```python
from build123d import *

# Parameters (mm, degrees)
F0_R     = 1.27
F1_DEPTH = 0.1


with BuildPart() as f1:
    # F0 (on Top) → F1 (new body)
    with BuildSketch(Plane.XY):
        with BuildLine():
            Line((0, 25.4), (0, 0))
            Line((0, 0), (44.45, 0))
            Line((44.45, 0), (88.9, 0))
            Line((88.9, 0), (88.9, 50.8))
            Line((88.9, 50.8), (57.15, 50.8))
            ThreePointArc((57.15, 50.8), (44.45, 44.45), (31.75, 50.8))
            Line((31.75, 50.8), (0, 50.8))
            Line((0, 50.8), (0, 25.4))
        make_face()
        with Locations((12.7, 9.525)):
            Circle(F0_R, mode=Mode.SUBTRACT)
        with BuildLine():
            ThreePointArc((13.97, 25.4), (12.7, 24.13), (11.43, 25.4))
            ThreePointArc((11.43, 25.4), (12.7, 26.67), (13.97, 25.4))
        make_face(mode=Mode.SUBTRACT)
        with Locations((31.75, 25.4)):
            Circle(F0_R, mode=Mode.SUBTRACT)
        with BuildLine():
            ThreePointArc((45.72, 12.7), (45.348026, 11.801974), (44.45, 11.43))
            ThreePointArc((44.45, 11.43), (43.551974, 13.598026), (45.72, 12.7))
        make_face(mode=Mode.SUBTRACT)
        with Locations((76.2, 9.525)):
            Circle(F0_R, mode=Mode.SUBTRACT)
        with Locations((44.45, 25.4)):
            Circle(F0_R, mode=Mode.SUBTRACT)
        with Locations((57.15, 25.4)):
            Circle(F0_R, mode=Mode.SUBTRACT)
        with Locations((76.2, 25.4)):
            Circle(F0_R, mode=Mode.SUBTRACT)
        with Locations((12.7, 41.275)):
            Circle(F0_R, mode=Mode.SUBTRACT)
        with Locations((44.45, 38.1)):
            Circle(F0_R, mode=Mode.SUBTRACT)
        with Locations((76.2, 41.275)):
            Circle(F0_R, mode=Mode.SUBTRACT)
    extrude(amount=F1_DEPTH)


solid = f1.part
```
Verification items for the finished model (mm, model axes). Round coordinates to 2 decimals unless told otherwise and drop trailing zeros. Order: outer loops, then holes, each group sorted by start corner. A loop starts at its lowest first (then second) coordinate and runs counter-clockwise, first axis right, second up.
1) Cross-section at B-B, the plane x = 76.2. Record the cut outline in (y, z) (3 decimals), plus the area to 3 significant figures.
Geometry says:
outline: (0, 0) - (8.255, 0) - (8.255, 0.1) - (0, 0.1) - close; (10.795, 0) - (24.13, 0) - (24.13, 0.1) - (10.795, 0.1) - close; (26.67, 0) - (40.005, 0) - (40.005, 0.1) - (26.67, 0.1) - close; (42.545, 0) - (50.8, 0) - (50.8, 0.1) - (42.545, 0.1) - close
area: 4.32 mm2
2) Material ranges on line 1 (X direction, y = 9, z = 0.05); line 2 (X direction, y = 46, z = 0.05), recorded low to high.
Geometry says:
line 1: x = 0 to 11.54, 13.86 to 75.04, 77.36 to 88.9
line 2: x = 0 to 37.61, 51.29 to 88.9
3) Cross-section at C-C, the plane x = 53. Record the cut outline in (y, z), plus the area to 3 significant figures.
Geometry says:
outline: (0, 0) - (46.95, 0) - (46.95, 0.1) - (0, 0.1) - close
area: 4.69 mm2
4) Depth check by flat-ended pin: pin 1 (1.5 mm diameter, centred on x = 44.45, y = 38.1, fed in from -Z). Enter the tip coordinate at first touch or a pass-through.
Geometry says:
pin 1: passes through
5) Cross-section at A-A, the plane y = 25.4. Record the cut outline in (x, z), plus the area to 3 significant figures.
Geometry says:
outline: (0, 0) - (11.43, 0) - (11.43, 0.1) - (0, 0.1) - close; (13.97, 0) - (30.48, 0) - (30.48, 0.1) - (13.97, 0.1) - close; (33.02, 0) - (43.18, 0) - (43.18, 0.1) - (33.02, 0.1) - close; (45.72, 0) - (55.88, 0) - (55.88, 0.1) - (45.72, 0.1) - close; (58.42, 0) - (74.93, 0) - (74.93, 0.1) - (58.42, 0.1) - close; (77.47, 0) - (88.9, 0) - (88.9, 0.1) - (77.47, 0.1) - close
area: 7.62 mm2
